Autodesk Inventor part; units mm, degrees
ref_plane "YZ Plane" through (0, 0, 0) normal (1, 0, 0) x (0, 1, 0)
ref_plane "XZ Plane" through (0, 0, 0) normal (0, 1, 0) x (-1, 0, 0)
ref_plane "XY Plane" through (0, 0, 0) normal (0, 0, 1) x (1, 0, 0)
sketch "Sketch1" plane through (0, 0, 0) normal (0, 1, 0) x (-1, 0, 0)
  line L0 (69.0976, -38.7621) -> (24.6476, -38.7621)
  line L1 (69.0976, -13.3621) -> (69.0976, -38.7621)
  line L2 (24.6476, -38.7621) -> (41.922, -38.7621)
  line L3 (37.3476, 43.7879) -> (24.6476, 43.7879)
  line L4 (69.0976, -13.3621) -> (37.3476, -13.3621)
  line L5 (37.3476, -13.3621) -> (37.3476, 43.7879)
  line L6 (-19.8024, -38.7621) -> (24.6476, -38.7621)
  line L7 (-19.8024, -13.3621) -> (-19.8024, -38.7621)
  line L8 (24.6476, -38.7621) -> (7.3732, -38.7621)
  line L9 (11.9476, 43.7879) -> (24.6476, 43.7879)
  line L10 (-19.8024, -13.3621) -> (11.9476, -13.3621)
  line L11 (11.9476, -13.3621) -> (11.9476, 43.7879)
  point P0 (0, 0)
  dimension "d0" = 44.45
  dimension "d1" = 12.7
  dimension "d2" = 25.4
  dimension "d3" = 82.55
extrude "Extrusion1" add sketch "Sketch1" along normal blind 2.286
sketch "Sketch2" plane through (0, 2.286, 0) normal (0, 1, 0) x (1, 0, 0)
  circle A0 centre (-24.6476, 26.0621) radius 2.0828
  line L0 (19.8024, 38.7621) -> (-69.0976, 38.7621)
  line L1 (19.8024, 13.3621) -> (19.8024, 38.7621)
  point P0 (0, 0)
  dimension "d6" = 4.1656
  dimension "d7" = 12.7
  dimension "d8" = 44.45
extrude "Extrusion2" cut sketch "Sketch2" against normal blind 2.286
pattern_linear "Rectangular Pattern1" count 4 spacing 12.7 along (1, 0, 0) count 4 spacing 12.7 along (-1, 0, 0) of "Extrusion2"
pattern_linear "Rectangular Pattern2" count 6 spacing 12.7 along (0, 0, 1) of "Extrusion2"
chamfer "Chamfer1" distance 2.54 angle 45 6 edges at (-69.0976, 1.143, -13.3621) (-37.3476, 1.143, 43.7879) (-11.9476, 1.143, 43.7879) (19.8024, 1.143, -13.3621) (19.8024, 1.143, -38.7621) (-69.0976, 1.143, -38.7621)
fillet "Fillet1" radius 3.175 2 edges at (-37.3476, 1.143, -13.3621) (-11.9476, 1.143, -13.3621)
properties part number "TGusset Versa"
For this review, take the finished solid that the model builds, in its own axes (mm). Round coordinates to 2 decimals unless told otherwise and drop trailing zeros. Write each loop counter-clockwise with the first axis right and the second up, starting at its lowest first coordinate (ties: lowest second). Pieces come first, ordered by that corner, then holes. Notation, with made-up numbers: (-17.75, -34) -> (18.25, -34) arc R16 ccw to (18.25, -25) -> close; hole circle Ø2 at (27, 12.5). An arc over 180 degrees is marked (long way). One line per question, with ' | ' between items. Start each with the question number.
(1) Add section C-C, the plane x = 5.5. Write out the cut boundary in (y, z).
(2) Add section B-B, the plane y = 0.9. Give the number of separate pieces and of enclosed holes in the cut face, plus the area to 3 significant figures.
(3) For line 1 along X through (y, z) = (0.4, -0.5); line 2 along Z through (x, y) = (7, 0.85); line 3 along X through (y, z) = (1.65, 31.5), list the stretches that pass through material, from the lowest coordinate up. Write a range as from..to.
(4) Add section A-A, the plane x = -49.5. Write out the cut boundary in (y, z), plus the area to 3 significant figures.
(5) Insertion check: P1, Ø2.5, axis at x = -37.35, z = -26.06, coming from the +Y side; P2, Ø1.1, axis at x = -50.5, y = 1, coming from the +Z side; P3, Ø0.7, axis at y = 1, z = 15.5, coming from the -X side. Each pin has a flat end and moves straight along its axis. Give the tip position at first contact, or say it passes through.
(6) Add section D-D, the plane z = 3.5. Write out the cut boundary in (x, y).
(7) Mouldability with a two-part tool opening along X and no side actions: class faces 1 (the face through (-22.724, 1.159, 25.536)), 2 (the face through (4, 1, -13.362)), 3 (the face through (19.802, 1, -26)) as released by +X, released by -X, zero draft, split by the parting line, or undercut.
Answer list:
1) outline: (0, -38.76) -> (2.29, -38.76) -> (2.29, -13.36) -> (0, -13.36) -> close
2) separate pieces: 1 | enclosed holes: 12 | area: 3,530 mm²
3) line 1: -37.35..-26.72, -22.57..-11.95 | line 2: -38.76..-13.36 | line 3: -37.35..-11.95
4) outline: (0, -38.76) -> (2.29, -38.76) -> (2.29, -28.07) -> (0, -28.07) -> close; (0, -24.05) -> (2.29, -24.05) -> (2.29, -13.36) -> (0, -13.36) -> close | area: 48.9 mm²
5) P1: through | P2: z = -13.36 | P3: x = -37.35
6) outline: (-37.35, 0) -> (-11.95, 0) -> (-11.95, 2.29) -> (-37.35, 2.29) -> close
7) face 1: undercut | face 2: zero draft | face 3: released by +X
